from build123d import *

# Parameters (mm, degrees)
BOSS_EXTRUDE1_DEPTH = 2.5
SKETCH2_R           = 1.5
CUT_EXTRUDE1_DEPTH  = 106.920143167
SKETCH4_W           = 15
SKETCH4_H           = 2
CUT_EXTRUDE2_DEPTH  = 2.5


with BuildPart() as part:
    # Sketch1 → Boss-Extrude1 (new body)
    with BuildSketch(Plane(origin=(0, 0, 0), x_dir=(1, 0, 0), z_dir=(0, 1, 0))):
        with BuildLine():
            Line((45.546700959, 65), (45.546700959, 49.998256331))
            ThreePointArc((45.546700959, 49.998256331), (44.082234865, 46.462722425), (40.546700959, 44.998256331))
            Line((40.546700959, 44.998256331), (-29.453299041, 44.998256331))
            ThreePointArc((-29.453299041, 44.998256331), (-32.988832947, 43.533790237), (-34.453299041, 39.998256331))
            Line((-34.453299041, 39.998256331), (-34.453299041, 31.248256331))
            Line((-34.453299041, 31.248256331), (-44.453299041, 31.248256331))
            Line((-44.453299041, 31.248256331), (-44.453299041, 46.248256331))
            Line((-44.453299041, 46.248256331), (-44.453299041, 60))
            ThreePointArc((-44.453299041, 60), (-45.917765135, 63.535533906), (-49.453299041, 65))
            Line((-49.453299041, 65), (-74.453299041, 65))
            ThreePointArc((-74.453299041, 65), (-77.988832947, 63.535533906), (-79.453299041, 60))
            Line((-79.453299041, 60), (-79.453299041, -60))
            ThreePointArc((-79.453299041, -60), (-77.988832947, -63.535533906), (-74.453299041, -65))
            Line((-74.453299041, -65), (-49.453299041, -65))
            ThreePointArc((-49.453299041, -65), (-45.917765135, -63.535533906), (-44.453299041, -60))
            Line((-44.453299041, -60), (-44.453299041, -46.251743669))
            Line((-44.453299041, -46.251743669), (-44.453299041, -31.251743669))
            Line((-44.453299041, -31.251743669), (-34.453299041, -31.251743669))
            Line((-34.453299041, -31.251743669), (-34.453299041, -40.001743669))
            ThreePointArc((-34.453299041, -40.001743669), (-32.988832947, -43.537277575), (-29.453299041, -45.001743669))
            Line((-29.453299041, -45.001743669), (40.546700959, -45.001743669))
            ThreePointArc((40.546700959, -45.001743669), (44.082234865, -46.466209763), (45.546700959, -50.001743669))
            Line((45.546700959, -50.001743669), (45.546700959, -65))
            ThreePointArc((45.546700959, -65), (47.011167053, -68.535533906), (50.546700959, -70))
            Line((50.546700959, -70), (70.546700959, -70))
            ThreePointArc((70.546700959, -70), (74.082234865, -68.535533906), (75.546700959, -65))
            Line((75.546700959, -65), (75.546700959, 65))
            ThreePointArc((75.546700959, 65), (74.082234865, 68.535533906), (70.546700959, 70))
            Line((70.546700959, 70), (50.546700959, 70))
            ThreePointArc((50.546700959, 70), (47.011167053, 68.535533906), (45.546700959, 65))
        make_face()
        with BuildLine():
            Line((-71.953299041, 60), (-66.953299041, 60))
            ThreePointArc((-66.953299041, 60), (-65.185532088, 59.267766953), (-64.453299041, 57.5))
            Line((-64.453299041, 57.5), (-64.453299041, -57.5))
            ThreePointArc((-64.453299041, -57.5), (-65.185532088, -59.267766953), (-66.953299041, -60))
            Line((-66.953299041, -60), (-71.953299041, -60))
            ThreePointArc((-71.953299041, -60), (-73.721065994, -59.267766953), (-74.453299041, -57.5))
            Line((-74.453299041, -57.5), (-74.453299041, 57.5))
            ThreePointArc((-74.453299041, 57.5), (-73.721065994, 59.267766953), (-71.953299041, 60))
        make_face(mode=Mode.SUBTRACT)
    extrude(amount=BOSS_EXTRUDE1_DEPTH)

    # Sketch2 → Cut-Extrude1 (cut, through all)
    with BuildSketch(Plane(origin=(0, 2.5, 0), x_dir=(1, 0, 0), z_dir=(0, 1, 0))):
        with Locations(Location((51.417773874, 27.5, 0), (0, 0, 270))):
            Circle(SKETCH2_R)
        with Locations(Location((51.417773874, -27.5, 0), (0, 0, 270))):
            Circle(SKETCH2_R)
        with Locations(Location((71.417773874, -27.5, 0), (0, 0, 270))):
            Circle(SKETCH2_R)
        with Locations(Location((71.417773874, 27.5, 0), (0, 0, 270))):
            Circle(SKETCH2_R)
    extrude(amount=-CUT_EXTRUDE1_DEPTH, mode=Mode.SUBTRACT)

    # Sketch4 → Cut-Extrude2 (cut)
    with BuildSketch(Plane.XZ):
        with Locations((62.046700959, -48.5)):
            Rectangle(SKETCH4_W, SKETCH4_H)
        with Locations((62.046700959, 48.5)):
            Rectangle(SKETCH4_W, SKETCH4_H)
    extrude(amount=-CUT_EXTRUDE2_DEPTH, mode=Mode.SUBTRACT)


solid = part.part
For this review, take the finished solid that the model builds, in its own axes (mm). A direction names the side the tool comes from. Round coordinates to 2 decimals unless told otherwise and drop trailing zeros. Loops run counter-clockwise (first coordinate to the right, second up) from the corner with the lowest first, then second, coordinate; pieces in that order, holes last. Notation, with made-up numbers: (79, -32) - (114, -32) arc R24 cw to (114, 1) - close; hole circle Ø11 at (-20.5, 27.5). An arc over 180 degrees is marked (long way). One line per item, written item: value. Start each with the question number.
Item 1: Take a section at B-B (x = 58.5). Give the boundary of the cut face in (y, z).
Item 2: Take a section at C-C (z = -10). Give the boundary of the cut face in (x, y), plus the area to 4 significant figures.
Item 3: For faces 4 (the cylindrical face through (-45.957, 1.232, 63.574)), 5 (the cylindrical face through (-45.88, 1.23, -63.5)), 6 (the flat face through (-3, 2.5, -1)), list the 3-axis set-ups (+Z, -Z, +X, -X, +Y, -Y) from which the entire face can be reached by the end or side of a thin tool; tool diameter is ignored.
Item 4: Take a section at A-A (z = -52.5). Give the boundary of the cut face in (x, y), plus the area to 4 significant figures.
Item 5: For L1, parallel to X at y = 1.2, z = -27.5; L2, parallel to X at y = 1.9, z = -33.5; L3, parallel to Z at x = 65, y = 0.1, list the stretches that pass through material, from the lowest coordinate up.
Item 6: The part is to be moulded in two halves that separate along X. For faces 1 (the cylindrical face through (74.12, 1.23, -68.5)), 2 (the cylindrical face through (47.05, 1.232, -68.574)), 3 (the cylindrical face through (44.12, 1.23, -46.5)), say which applies: +X half, -X half, draft (parallel to the pull), parting line (faces both ways), or undercut.
Item 7: Clearance check with flat-ended pins moving along their axes: pin 1 Ø12 at (x, z) = (1.5, 52.5) entering from +Y; pin 2 Ø1.2 at (x, y) = (0, 1) entering from -Z; pin 3 Ø1.2 at (x, y) = (0, 1.5) entering from +Z. State where each tip first meets the part, or that it passes through.
Item 8: Take a section at D-D (x = 20.5). Give the boundary of the cut face in (y, z).
Answer below:
1. outline: (0, -70) - (2.5, -70) - (2.5, -49.5) - (0, -49.5) - close; (0, -47.5) - (2.5, -47.5) - (2.5, 47.5) - (0, 47.5) - close; (0, 49.5) - (2.5, 49.5) - (2.5, 70) - (0, 70) - close
2. outline: (-79.45, 0) - (-74.45, 0) - (-74.45, 2.5) - (-79.45, 2.5) - close; (-64.45, 0) - (75.55, 0) - (75.55, 2.5) - (-64.45, 2.5) - close
2. area: 362.5 mm2
3. face 4: +Z, +Y, -Y
3. face 5: -Z, +Y, -Y
3. face 6: +Z, -Z, +X, -X, +Y
4. outline: (-79.45, 0) - (-74.45, 0) - (-74.45, 2.5) - (-79.45, 2.5) - close; (-64.45, 0) - (-44.45, 0) - (-44.45, 2.5) - (-64.45, 2.5) - close; (45.55, 0) - (75.55, 0) - (75.55, 2.5) - (45.55, 2.5) - close
4. area: 137.5 mm2
5. L1: x = -79.45 to -74.45, -64.45 to 49.92, 52.92 to 69.92, 72.92 to 75.55
5. L2: x = -79.45 to -74.45, -64.45 to -44.45, -34.45 to 75.55
5. L3: z = -70 to -49.5, -47.5 to 47.5, 49.5 to 70
6. face 1: +X half
6. face 2: -X half
6. face 3: undercut
7. pin 1: passes through
7. pin 2: stops at z = -45
7. pin 3: stops at z = 45
8. outline: (0, -45) - (2.5, -45) - (2.5, 45) - (0, 45) - close
